from build123d import *

# Parameters (mm, degrees)
F1_DEPTH = 2.5


with BuildPart() as f1:
    # F0 (on Top) → F1 (new body)
    with BuildSketch(Plane.XY):
        with BuildLine():
            ThreePointArc((13.64249, 9.534957), (0, 8.599999), (-13.64249, 9.534957))
            ThreePointArc((-13.64249, 9.534957), (-14.152097, 9.274517), (-14.083427, 8.706351))
            Line((-14.083427, 8.706351), (-3.5, -3.129614))
            ThreePointArc((-3.5, -3.129614), (0, -4.695155), (3.5, -3.129614))
            Line((3.5, -3.129614), (14.083427, 8.706351))
            ThreePointArc((14.083427, 8.706351), (14.152097, 9.274517), (13.64249, 9.534957))
        make_face()
        with BuildLine():
            ThreePointArc((-1.6, 5), (1e-06, 6.599999), (1.6, 4.999999))
            Line((1.6, 4.999999), (1.6, -1e-06))
            ThreePointArc((1.6, -1e-06), (-1e-06, -1.6), (-1.6, 0))
            Line((-1.6, 0), (-1.6, 5))
        make_face(mode=Mode.SUBTRACT)
    extrude(amount=F1_DEPTH)


solid = f1.part
Geometry: final body of the model. Coordinates: model frame, mm. A direction names the side the tool comes from. Coordinates: 2 decimals unless noted, no trailing zeros. Loops run counter-clockwise (first coordinate to the right, second up) from the corner with the lowest first, then second, coordinate; pieces in that order, holes last. Notation, with made-up numbers: M -30,-10 L 24,-10 A21 cw 24,13 Z; hole C 76,17 d11. An arc over 180 degrees is marked long. One line per item, written item: value. Start each with the question number.
1) Material intervals for L1, parallel to X at y = 3.5, z = 2.4; L2, parallel to X at y = 2.5, z = 1.35; L3, parallel to X at y = -3.75, z = 0.4, sorted ascending. Write a range as from..to.
2) Cut plane C-C (x = -9.5). Return loops of the section in (y, z), then the cut area to 3 significant figures.
3) Draft query along X for faces 1 (the cylindrical face through (-0.055, -4.695, 1.232)), 2 (the cylindrical face through (0, -1.6, 1.2)), 3 (the flat face through (8.72, 2.71, 1.23)), 4 (the flat face through (-1.6, 2, 1)). Return one class per face: released by +X, released by -X, zero draft, split by the parting line, or undercut.
4) Cut plane A-A (x = 0). Return loops of the section in (y, z), then the cut area to 3 significant figures.
5) Reachability of faces 5 (the flat face through (1.6, 3, 1)), 6 (the flat face through (3, 4, 2.5)) from +Z, -Z, +X, -X, +Y, -Y: full face, straight path, thin tool, end or side. Return the list, or none.
6) Pin query (flat end, axial travel): P1, Ø1.5, axis at x = 6.5, z = 1.5, coming from the -Y side; P2, Ø1, axis at x = -2.5, z = 2, coming from the +Y side (3 decimals); P3, Ø1, axis at y = -1.5, z = 2, coming from the -X side. Return the tip coordinate at first contact, or that it passes through.
7) Cut plane B-B (z = 0.55). Return loops of the section in (x, y).
8) Cut plane D-D (y = 7.25). Return loops of the section in (x, z), then the cut area to 3 significant figures.
Evaluation:
1. L1: -9.43..-1.6, 1.6..9.43
1. L2: -8.53..-1.6, 1.6..8.53
1. L3: -2.83..2.83
2. outline: M 3.58,0 L 9.05,0 L 9.05,2.5 L 3.58,2.5 Z
2. area: 13.7 mm^2
3. face 1: split by the parting line
3. face 2: undercut
3. face 3: released by +X
3. face 4: undercut
4. outline: M -4.7,0 L -1.6,0 L -1.6,2.5 L -4.7,2.5 Z; M 6.6,0 L 8.6,0 L 8.6,2.5 L 6.6,2.5 Z
4. area: 12.7 mm^2
5. face 5: +Z, -Z
5. face 6: +Z, +X, -X, +Y, -Y
6. P1: y = -0.61
6. P2: y = 8.645
6. P3: x = -5.4
7. outline: M -14.08,8.71 L -3.5,-3.13 A4.7 ccw 3.5,-3.13 L 14.08,8.71 A0.5 ccw 13.64,9.53 A100 cw -13.64,9.53 A0.5 ccw Z; hole M -1.6,0 A1.6 ccw 1.6,0 L 1.6,5 A1.6 ccw -1.6,5 Z
8. outline: M -12.78,0 L 12.78,0 L 12.78,2.5 L -12.78,2.5 Z
8. area: 63.9 mm^2
